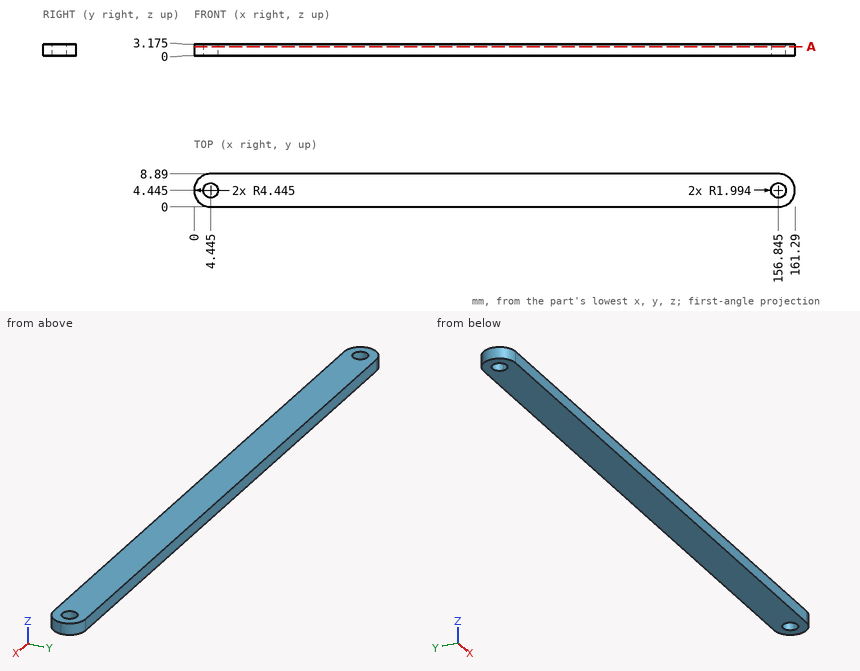
For this review, use the dimensioned drawing (mm, ordinates from the lowest corner) and the shaded views. Coordinates: 2 decimals unless noted, no trailing zeros. Loops run counter-clockwise (first coordinate to the right, second up) from the corner with the lowest first, then second, coordinate; pieces in that order, holes last. Notation, with made-up numbers: (-34, 29.5) -> (-19, 29.5) arc R17 ccw to (-19, 49.5) -> close; hole circle Ø1 at (51.5, 29.25). An arc over 180 degrees is marked (long way). Write each question's results on one line, items separated by ' | '.
Q1. Add section A-A, the plane z = 2.45. State the section outline as (x, y) points (3 decimals), then the cut area to 3 significant figures.
Taken from the geometry:
outline: (4.445, 0) -> (156.845, 0) arc R4.445 ccw to (156.845, 8.89) -> (4.445, 8.89) arc R4.445 ccw to start; hole circle Ø3.988 at (4.445, 4.445); hole circle Ø3.988 at (156.845, 4.445) | area: 1,390 mm²
Q2. To check wall thickness, follow line 1 along X through (y, z) = (4.5, 3); line 2 along X through (y, z) = (3.75, 1) (1 decimal); line 3 along X through (y, z) = (7.5, 1.1). State the ranges of each line that lie inside material, in increasing order. Write a range as [from, to].
Taken from the geometry:
line 1: [0, 2.45], [6.44, 154.85], [158.84, 161.29] | line 2: [0.1, 2.6], [6.3, 155], [158.7, 161.2] | line 3: [1.22, 160.07]
Q3. For pin 1 Ø1 at (y, z) = (5, 0.5) entering from +X, flat-tipped, find the tip position at first contact; note if it passes through.
Taken from the geometry:
pin 1: x = 161.29
